Build history of the part. All positions in model axes, mm. A direction names the side the tool comes from. Coordinates: 2 decimals unless noted, no trailing zeros. Order: outer loops, then holes, each group sorted by start corner. A loop starts at its lowest first (then second) coordinate and runs counter-clockwise, first axis right, second up. Notation, with made-up numbers: (61.25, 38.5) - (86.25, 38.5) arc R32 ccw to (86.25, 69.5) - close; hole circle Ø8 at (26, -37.75). An arc over 180 degrees is marked (long way). One line per item, written item: value.
from build123d import *

# Parameters (mm, degrees)
F0_R     = 3.25
F1_DEPTH = 4.5


# Not quite as in the source:
# - ends of sketch curves that miss each other by under 0.0002 mm in the source are joined


with BuildPart() as f1:
    # F0 (on Front) → F1 (new body)
    with BuildSketch(Plane.XZ):
        with BuildLine():
            ThreePointArc((-6.3848473051, 0.378745021), (-6.458741388, 0.201395137), (-6.6250810223, 0.1052471112))
            Line((-6.6250810223, 0.1052471112), (-7.499995, -0.070416))
            Line((-7.499995, -0.070416), (-8.481787, -0.617539))
            ThreePointArc((-8.481787, -0.617539), (-8.4534361937, -0.9498951475), (-8.4120672698, -1.2808810391))
            Line((-8.4120672698, -1.2808810391), (-7.337975, -1.611925))
            Line((-7.337975, -1.611925), (-6.445659, -1.601845))
            ThreePointArc((-6.445659, -1.601845), (-6.2629631412, -1.6613077046), (-6.1538101366, -1.819419039))
            ThreePointArc((-6.1538101366, -1.819419039), (-6.0867618577, -2.039112292), (-6.0118718389, -2.2562609412))
            ThreePointArc((-6.0118718389, -2.2562609412), (-6.0072434399, -2.4483319562), (-6.120095855, -2.6038242044))
            Line((-6.120095855, -2.6038242044), (-6.84792, -3.12016))
            Line((-6.84792, -3.12016), (-7.522298, -4.019312))
            ThreePointArc((-7.522298, -4.019312), (-7.3612165371, -4.3114029523), (-7.1888002117, -4.5969471336))
            Line((-7.1888002117, -4.5969471336), (-6.07292, -4.462499))
            Line((-6.07292, -4.462499), (-5.261849, -4.090353))
            ThreePointArc((-5.261849, -4.090353), (-5.0707630565, -4.0703658396), (-4.9067374821, -4.1704104038))
            ThreePointArc((-4.9067374821, -4.1704104038), (-4.7561274158, -4.343839289), (-4.5993898038, -4.5117538102))
            ThreePointArc((-4.5993898038, -4.5117538102), (-4.5170386347, -4.6853377004), (-4.5568904277, -4.8732883391))
            Line((-4.5568904277, -4.8732883391), (-5.011778, -5.641017))
            Line((-5.011778, -5.641017), (-5.262135, -6.736727))
            ThreePointArc((-5.262135, -6.736727), (-4.9961722078, -6.9380502226), (-4.7225170454, -7.128782068))
            Line((-4.7225170454, -7.128782068), (-3.757802, -6.552084))
            Line((-3.757802, -6.552084), (-3.168217, -5.882218))
            ThreePointArc((-3.168217, -5.882218), (-3.0017803181, -5.7862379026), (-2.8112432041, -5.8109184175))
            ThreePointArc((-2.8112432041, -5.8109184175), (-2.6031126369, -5.9080957654), (-2.3916319825, -5.9977409564))
            ThreePointArc((-2.3916319825, -5.9977409564), (-2.2457975094, -6.1228225948), (-2.2057577098, -6.3107329173))
            Line((-2.2057577098, -6.3107329173), (-2.309055, -7.197108))
            Line((-2.309055, -7.197108), (-2.092101, -8.299918))
            ThreePointArc((-2.092101, -8.299918), (-1.7672462291, -8.3756592743), (-1.4396719873, -8.4385959262))
            Line((-1.4396719873, -8.4385959262), (-0.792926, -7.519371))
            Line((-0.792926, -7.519371), (-0.526772, -6.667613))
            ThreePointArc((-0.526772, -6.667613), (-0.4137637804, -6.5122339125), (-0.2296610073, -6.457282204))
            ThreePointArc((-0.2296610073, -6.457282204), (2.4984e-06, -6.461404), (0.229662, -6.457281998))
            ThreePointArc((0.229662, -6.457281998), (0.4137637804, -6.5122339125), (0.5267720218, -6.6676129932))
            Line((0.5267720218, -6.6676129932), (0.792926, -7.519371))
            Line((0.792926, -7.519371), (1.439676, -8.438595))
            ThreePointArc((1.439676, -8.438595), (1.7672522889, -8.3756579862), (2.0921050032, -8.2999170124))
            Line((2.0921050032, -8.2999170124), (2.309055, -7.197108))
            Line((2.309055, -7.197108), (2.205757, -6.310733))
            ThreePointArc((2.205757, -6.310733), (2.2457975094, -6.1228225948), (2.3916327595, -5.9977404031))
            ThreePointArc((2.3916327595, -5.9977404031), (2.6031159206, -5.9080943034), (2.8112438605, -5.8109177148))
            ThreePointArc((2.8112438605, -5.8109177148), (3.0017803181, -5.7862379026), (3.1682168748, -5.8822191102))
            Line((3.1682168748, -5.8822191102), (3.757802, -6.552084))
            Line((3.757802, -6.552084), (4.72252, -7.12878))
            ThreePointArc((4.72252, -7.12878), (4.9961769033, -6.9380468111), (5.2621377529, -6.7367246866))
            Line((5.2621377529, -6.7367246866), (5.011778, -5.641017))
            Line((5.011778, -5.641017), (4.556891, -4.873288))
            ThreePointArc((4.556891, -4.873288), (4.5170386766, -4.6853373435), (4.599391221, -4.5117522139))
            ThreePointArc((4.599391221, -4.5117522139), (4.7561281073, -4.3438385211), (4.9067371021, -4.1704100855))
            ThreePointArc((4.9067371021, -4.1704100855), (5.0707626825, -4.0703659239), (5.2618489304, -4.0903531516))
            Line((5.2618489304, -4.0903531516), (6.07292, -4.462499))
            Line((6.07292, -4.462499), (7.188798, -4.596951))
            ThreePointArc((7.188798, -4.596951), (7.361216975, -4.3114021938), (7.5222993001, -4.0193091579))
            Line((7.5222993001, -4.0193091579), (6.84792, -3.12016))
            Line((6.84792, -3.12016), (6.120096, -2.603824))
            ThreePointArc((6.120096, -2.603824), (6.0072434399, -2.4483319562), (6.0118725915, -2.2562588509))
            ThreePointArc((6.0118725915, -2.2562588509), (6.0867621941, -2.0391112566), (6.153810771, -1.8194179346))
            ThreePointArc((6.153810771, -1.8194179346), (6.2629631412, -1.6613077046), (6.4456589984, -1.6018451428))
            Line((6.4456589984, -1.6018451428), (7.337975, -1.611925))
            Line((7.337975, -1.611925), (8.412067, -1.280885))
            ThreePointArc((8.412067, -1.280885), (8.4534363514, -0.9498936467), (8.481787446, -0.6175350292))
            Line((8.481787446, -0.6175350292), (7.499995, -0.070416))
            Line((7.499995, -0.070416), (6.625082, 0.105247))
            ThreePointArc((6.625082, 0.105247), (6.4587417115, 0.2013947687), (6.3848473051, 0.378745021))
            ThreePointArc((6.3848473051, 0.378745021), (6.3649400086, 0.6075793237), (6.3368346677, 0.835549953))
            ThreePointArc((6.3368346677, 0.835549953), (6.3722414368, 1.0243877393), (6.5149571212, 1.1530187192))
            Line((6.5149571212, 1.1530187192), (7.334228, 1.506748))
            Line((7.334228, 1.506748), (8.180813, 2.246041))
            ThreePointArc((8.180813, 2.246041), (8.0839798549, 2.5652420945), (7.974697483, 2.8803981782))
            Line((7.974697483, 2.8803981782), (6.855252, 2.980885))
            Line((6.855252, 2.980885), (5.98453, 2.785503))
            ThreePointArc((5.98453, 2.785503), (5.7934636286, 2.8056817814), (5.6538228924, 2.9376439429))
            ThreePointArc((5.6538228924, 2.9376439429), (5.5425619412, 3.1385971137), (5.4241623811, 3.3354272386))
            ThreePointArc((5.4241623811, 3.3354272386), (5.3797004129, 3.5223406923), (5.4577587633, 3.697898218))
            Line((5.4577587633, 3.697898218), (6.062326, 4.354273))
            Line((6.062326, 4.354273), (6.535022, 5.373988))
            ThreePointArc((6.535022, 5.373988), (6.3167298633, 5.6262074349), (6.088709809, 5.8696678139))
            Line((6.088709809, 5.8696678139), (5.025173, 5.506148))
            Line((5.025173, 5.506148), (4.309199, 4.973502))
            ThreePointArc((4.309199, 4.973502), (4.1264437672, 4.9142226849), (3.9452018311, 4.9779787843))
            ThreePointArc((3.9452018311, 4.9779787843), (3.7618245482, 5.1163055389), (3.5736032135, 5.2479613173))
            ThreePointArc((3.5736032135, 5.2479613173), (3.4569607105, 5.4006300799), (3.4568644648, 5.5927591806))
            Line((3.4568644648, 5.5927591806), (3.742192, 6.438288))
            Line((3.742192, 6.438288), (3.759267, 7.562107))
            ThreePointArc((3.759267, 7.562107), (3.4572596135, 7.7037332148), (3.1499290285, 7.8334010714))
            Line((3.1499290285, 7.8334010714), (2.326197, 7.06873))
            Line((2.326197, 7.06873), (1.888768, 6.290921))
            ThreePointArc((1.888768, 6.290921), (1.7459243673, 6.1624334899), (1.554419964, 6.1469598562))
            ThreePointArc((1.554419964, 6.1469598562), (1.3306339934, 6.1987408207), (1.1051359772, 6.2424578697))
            ThreePointArc((1.1051359772, 6.2424578697), (0.9364810051, 6.3344853457), (0.8582472195, 6.5099649269))
            Line((0.8582472195, 6.5099649269), (0.775, 7.398447))
            Line((0.775, 7.398447), (0.3335, 8.432051))
            ThreePointArc((0.3335, 8.432051), (-1.4988e-06, 8.438596), (-0.3335029952, 8.4320508773))
            Line((-0.3335029952, 8.4320508773), (-0.775, 7.398447))
            Line((-0.775, 7.398447), (-0.858248, 6.509965))
            ThreePointArc((-0.858248, 6.509965), (-0.9364806674, 6.3344857115), (-1.1051359033, 6.2424574482))
            ThreePointArc((-1.1051359033, 6.2424574482), (-1.3306359057, 6.1987404142), (-1.5544199034, 6.146959614))
            ThreePointArc((-1.5544199034, 6.146959614), (-1.7459243673, 6.1624334899), (-1.8887681854, 6.2909208957))
            Line((-1.8887681854, 6.2909208957), (-2.326197, 7.06873))
            Line((-2.326197, 7.06873), (-3.149932, 7.8334))
            ThreePointArc((-3.149932, 7.8334), (-3.4572626886, 7.7037318457), (-3.759269185, 7.5621053752))
            Line((-3.759269185, 7.5621053752), (-3.742192, 6.438288))
            Line((-3.742192, 6.438288), (-3.456865, 5.59276))
            ThreePointArc((-3.456865, 5.59276), (-3.4569605775, 5.4006304728), (-3.5736028777, 5.2479608182))
            ThreePointArc((-3.5736028777, 5.2479608182), (-3.7618263316, 5.1163042431), (-3.9452020076, 4.9779790098))
            ThreePointArc((-3.9452020076, 4.9779790098), (-4.1264437672, 4.9142226849), (-4.3091988413, 4.9735022134))
            Line((-4.3091988413, 4.9735022134), (-5.025173, 5.506148))
            Line((-5.025173, 5.506148), (-6.088712, 5.869665))
            ThreePointArc((-6.088712, 5.869665), (-6.3167319914, 5.6262050713), (-6.5350238583, 5.3739858822))
            Line((-6.5350238583, 5.3739858822), (-6.062326, 4.354273))
            Line((-6.062326, 4.354273), (-5.457759, 3.697898))
            ThreePointArc((-5.457759, 3.697898), (-5.3797004129, 3.5223406923), (-5.4241620701, 3.3354270439))
            ThreePointArc((-5.4241620701, 3.3354270439), (-5.5425631892, 3.1385949521), (-5.6538231778, 2.9376430943))
            ThreePointArc((-5.6538231778, 2.9376430943), (-5.7934636286, 2.8056817814), (-5.9845300103, 2.785502954))
            Line((-5.9845300103, 2.785502954), (-6.855252, 2.980885))
            Line((-6.855252, 2.980885), (-7.974699, 2.880395))
            ThreePointArc((-7.974699, 2.880395), (-8.0839806406, 2.5652396762), (-8.1808133092, 2.2460390872))
            Line((-8.1808133092, 2.2460390872), (-7.334228, 1.506748))
            Line((-7.334228, 1.506748), (-6.514956, 1.153019))
            ThreePointArc((-6.514956, 1.153019), (-6.3722414368, 1.0243877393), (-6.3368349167, 0.8355489882))
            ThreePointArc((-6.3368349167, 0.8355489882), (-6.3649402163, 0.6075773468), (-6.3848473051, 0.378745021))
        make_face()
        with Locations((0, -0.061404)):
            Circle(F0_R, mode=Mode.SUBTRACT)
    extrude(amount=F1_DEPTH)


solid = f1.part
1. Probe line 1 along Z through (x, y) = (0, -2.6); line 2 along X through (y, z) = (-1.4, 7.5); line 3 along Z through (x, y) = (7, -2.75). List the from-to ranges inside material, lowest first.
Values found:
line 1: z = -6.46 to -3.31, 3.19 to 8.44
line 2: x = -3.76 to -2.79, -0.73 to 0.73, 2.79 to 3.76
line 3: z = -4.57 to -3.32, -1.61 to 0.03, 1.36 to 2.97
2. Band-saw the part on B-B, the plane z = 2.5. Give the cut face in (x, y), and give its area (3 significant figures).
Values found:
outline: (-8.1, -4.5) - (-2, -4.5) - (-2, 0) - (-8.1, 0) - close; (2, -4.5) - (8.1, -4.5) - (8.1, 0) - (2, 0) - close
area: 54.9 mm2
3. Band-saw the part on A-A, the plane x = 0. Give the cut face in (y, z).
Values found:
outline: (-4.5, -6.46) - (0, -6.46) - (0, -3.31) - (-4.5, -3.31) - close; (-4.5, 3.19) - (0, 3.19) - (0, 8.44) - (-4.5, 8.44) - close
4. Two-plate mould, pull along Z, no slides. Class faces 1 (the face through (4.233, -2.218, -6.836)), 2 (the face through (2.744, -2.218, 7.456)), 3 (the face through (5.14, -2.22, -6.2)): pulls with the +Z half, pulls with the -Z half, needs draft (parallel to the pull), parting line crosses it, or undercut.
Values found:
face 1: pulls with the -Z half
face 2: pulls with the +Z half
face 3: undercut
5. 3-axis set-ups, long thin cutter, end or side, ignore diameter. For faces 4 (the face through (0.817, -2.218, 6.948)), 5 (the face through (-7.98, -2.22, -0.34)), 6 (the face through (8, -2.22, -0.35)), 7 (the face through (6.62, -2.22, -4.53)): which of +Z, -Z, +X, -X, +Y, -Y reach the whole face in a straight line?
Values found:
face 4: +Z, +Y, -Y
face 5: -X, +Y, -Y
face 6: +X, +Y, -Y
face 7: -Z, +Y, -Y
